Could you check a few things on this model? Use its own coordinates, in mm. Coordinates: 2 decimals unless noted, no trailing zeros. Loops run counter-clockwise (first coordinate to the right, second up) from the corner with the lowest first, then second, coordinate; pieces in that order, holes last. Notation, with made-up numbers: M -32,-18.75 L -7,-18.75 A18 cw -7,8.25 Z; hole C 73.5,-25.75 d2. An arc over 180 degrees is marked long. Return JSON: item names as keys, results as strings. Group by question number.
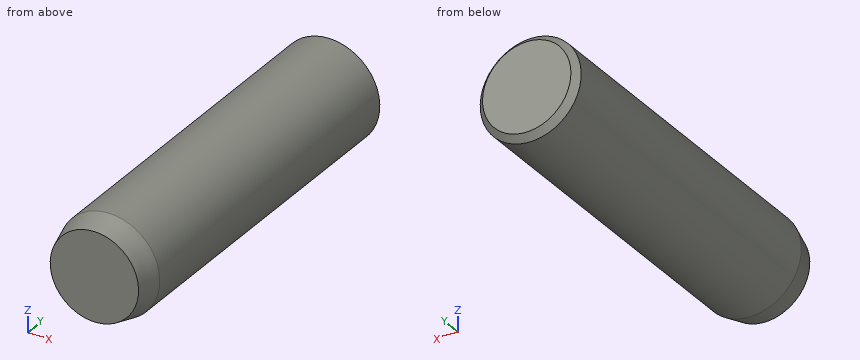
from build123d import *

# Parameters (mm, degrees)
SKETCH_1_R      = 4
EXTRUDE_1_DEPTH = 15
CHAMFER_1_SIZE  = 0.5
CHAMFER_2_SIZE  = 0.5
CHAMFER_2_SIZE2 = 1.866025404


with BuildPart() as part:
    # 草圖1 → 伸長1 (new, symmetric)
    with BuildSketch(Plane(origin=(0, 0, 0), x_dir=(1, 0, 0), z_dir=(0, 1, 0))):
        with Locations(Location((0, 0, 0), (0, 0, 270))):
            Circle(SKETCH_1_R)
    extrude(amount=EXTRUDE_1_DEPTH, both=True)

    # 導角1
    chamfer_1_edges = [part.edges().sort_by_distance(p)[0] for p in [
        (0, 15, -4),
    ]]
    chamfer(chamfer_1_edges, length=CHAMFER_1_SIZE)

    # 導角2
    chamfer_2_edges = [part.edges().sort_by_distance(p)[0] for p in [
        (0, -15, -4),
    ]]
    chamfer_2_side = [part.faces().sort_by_distance(p)[0] for p in [
        (0, -15, 0),
    ]]
    chamfer(chamfer_2_edges, length=CHAMFER_2_SIZE, length2=CHAMFER_2_SIZE2, reference=chamfer_2_side[0])


solid = part.part
(1) If I drill on L1, parallel to X at y = 4.5, z = 3.5; L2, parallel to X at y = -5.75, z = -2; L3, parallel to Z at x = -2.25, y = -11, over which ranges is the centre line in solid material (lowest first)? Write a range as [from, to].
(2) Imagine slicing it at A-A, the plane y = -1.25. Write out the boundary of the cut face in (x, z).
(3) Will this pin go through, and if not, where does the flat tip stop? P1, Ø1, axis at y = 7.5, z = -1.5, coming from the +X side.
Checks:
{
 "1": {"L1": "[-1.94, 1.94]", "L2": "[-3.46, 3.46]", "L3": "[-3.31, 3.31]"},
 "2": {"outline": "C 0,0 d8"},
 "3": {"P1": "x = 3.87"}
}
